Input: part model. Units: mm. Frame: model coordinates. Face numbers are marked on the shaded views. A direction names the side the tool comes from. Coordinates: 2 decimals unless noted, no trailing zeros. Loops run counter-clockwise (first coordinate to the right, second up) from the corner with the lowest first, then second, coordinate; pieces in that order, holes last. Notation, with made-up numbers: (56.5, 24.5) -> (72.5, 24.5) arc R19 ccw to (72.5, 48.5) -> close; hole circle Ø6 at (-39.5, -4). An arc over 180 degrees is marked (long way). Put each result on its own line as item: value. Start each with the question number.
1) Contact query for flat-ended pins moving along their axis: P1, Ø7, axis at x = 53.5, y = 8, coming from the -Z side; P2, Ø1.5, axis at y = 11, z = 55.5, coming from the -X side; P3, Ø1.5, axis at x = 3.5, y = 10.5, coming from the -Z side. Output: stop coordinate, or through.
2) Cut plane C-C (y = 18.75). Return the cut outline in (x, z).
3) Cut plane B-B (y = 5.5). Return the cut outline in (x, z).
4) Material intervals for L1, parallel to Z at x = -39, y = 3.25; L2, parallel to X at y = 15.25, z = 10; L3, parallel to X at y = 4, z = 65, sorted ascending.
5) Cut plane A-A (x = 50). Return the cut outline in (y, z).
6) Set-up query: the marked faces 1, 2 and 3. Return all of +Z, -Z, +X, -X, +Y, -Y with unobstructed straight access to the full face (end or side cutting, diameter ignored); none if empty.
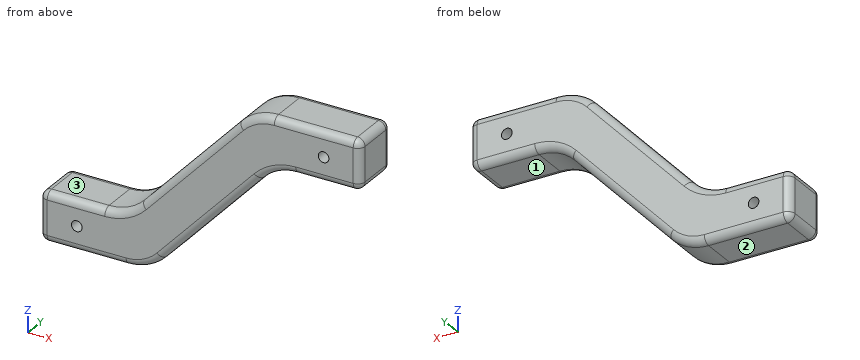
from build123d import *

# Parameters (mm, degrees)
CROQUIS1_R              = 2.15
SALIENTE_EXTRUIR1_DEPTH = 20
REDONDEO1_R             = 20
REDONDEO2_R             = 3


with BuildPart() as part:
    # Croquis1 → Saliente-Extruir1 (new body)
    with BuildSketch(Plane(origin=(0, 0, 0), x_dir=(1, 0, 0), z_dir=(0, 1, 0))):
        Polygon((-65, 0), (-21.305768696, 0), (30, -55), (65, -55), (65, -75), (21.305768696, -75), (-30, -20), (-65, -20), align=None)
        with Locations(Location((-50, -10, 0), (0, 0, 270))):
            Circle(CROQUIS1_R, mode=Mode.SUBTRACT)
        with Locations(Location((50, -65, 0), (0, 0, 270))):
            Circle(CROQUIS1_R, mode=Mode.SUBTRACT)
    extrude(amount=SALIENTE_EXTRUIR1_DEPTH)

    # Redondeo1
    redondeo1_edges = [part.edges().sort_by_distance(p)[0] for p in [
        (-21.305768696, 10, 0),
        (30, 10, 55),
        (21.305768696, 10, 75),
        (-30, 10, 20),
    ]]
    fillet(redondeo1_edges, radius=REDONDEO1_R)

    # Redondeo2
    redondeo2_edges = [part.edges().sort_by_distance(p)[0] for p in [
        (-51.847115652, 0, 20),
        (-65, 0, 10),
        (-65, 10, 0),
        (65, 10, 55),
        (65, 10, 75),
        (-65, 10, 20),
        (65, 20, 65),
        (51.847115652, 20, 55),
        (47.5, 0, 75),
        (47.5, 20, 75),
        (-47.5, 0, 0),
        (4.347115652, 0, 27.5),
        (-4.347115652, 0, 47.5),
        (-22.026573691, 0, 1.658122427),
        (22.026573691, 0, 73.341877573),
        (-4.347115652, 20, 47.5),
        (4.347115652, 20, 27.5),
        (-47.5, 20, 0),
        (-22.026573691, 20, 1.658122427),
        (22.026573691, 20, 73.341877573),
        (30.720804996, 0, 53.341877573),
        (30.720804996, 20, 53.341877573),
        (-30.720804996, 0, 21.658122427),
        (-30.720804996, 20, 21.658122427),
        (-65, 20, 10),
        (-51.847115652, 20, 20),
        (51.847115652, 0, 55),
        (65, 0, 65),
    ]]
    fillet(redondeo2_edges, radius=REDONDEO2_R)


solid = part.part
Results found:
1. P1: stops at z = 55
1. P2: stops at x = 2.42
1. P3: stops at z = 25.79
2. outline: (-64.44, 3) arc R2.44 ccw to (-62, 0.56) -> (-30, 0.56) arc R19.44 ccw to (-15.79, 6.74) -> (23.66, 49.03) arc R20.56 cw to (38.69, 55.56) -> (62, 55.56) arc R2.44 ccw to (64.44, 58) -> (64.44, 72) arc R2.44 ccw to (62, 74.44) -> (30, 74.44) arc R19.44 ccw to (15.79, 68.26) -> (-23.66, 25.97) arc R20.56 cw to (-38.69, 19.44) -> (-62, 19.44) arc R2.44 ccw to (-64.44, 17) -> close; hole circle Ø4.3 at (-50, 10); hole circle Ø4.3 at (50, 65)
3. outline: (-65, 3) arc R3 ccw to (-62, 0) -> (-30, 0) arc R20 ccw to (-15.38, 6.36) -> (24.07, 48.64) arc R20 cw to (38.69, 55) -> (62, 55) arc R3 ccw to (65, 58) -> (65, 72) arc R3 ccw to (62, 75) -> (30, 75) arc R20 ccw to (15.38, 68.64) -> (-24.07, 26.36) arc R20 cw to (-38.69, 20) -> (-62, 20) arc R3 ccw to (-65, 17) -> close; hole circle Ø4.3 at (-50, 10); hole circle Ø4.3 at (50, 65)
4. L1: z = 0 to 20
4. L2: x = -65 to -52.15, -47.85 to -11.98
4. L3: x = 11.98 to 47.85, 52.15 to 65
5. outline: (0, 58) arc R3 ccw to (3, 55) -> (17, 55) arc R3 ccw to (20, 58) -> (20, 62.85) -> (0, 62.85) -> close; (0, 67.15) -> (20, 67.15) -> (20, 72) arc R3 ccw to (17, 75) -> (3, 75) arc R3 ccw to (0, 72) -> close
6. face 1: -Z, +X, +Y, -Y
6. face 2: -Z, +X, -X, +Y, -Y
6. face 3: +Z, -X, +Y, -Y
